Read the model definition and answer for the solid it produces. Units are mm, in the model's axes. Face numbers are marked on the shaded views. A direction names the side the tool comes from. Coordinates: 2 decimals unless noted, no trailing zeros. Order: outer loops, then holes, each group sorted by start corner. A loop starts at its lowest first (then second) coordinate and runs counter-clockwise, first axis right, second up.
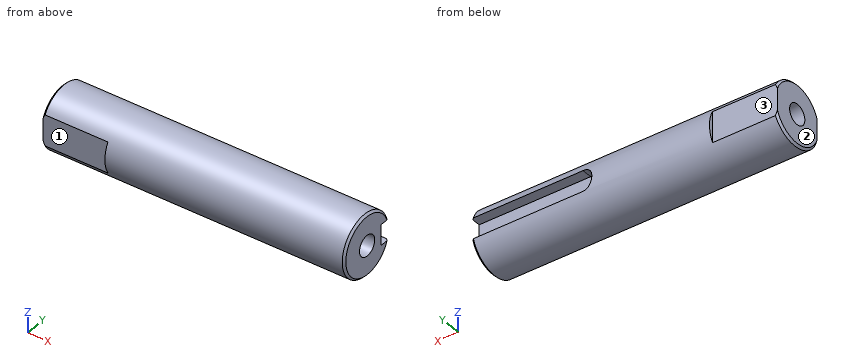
from build123d import *

# Parameters (mm, degrees)
SKETCH_2_W                     = 75
SKETCH_2_H                     = 7.5
CUT_EXTRUDE_START              = 4.5
CUT_EXTRUDE_1_DEPTH            = 72.246287038
CUT_EXTRUDE_2_DEPTH            = 76.746287157
CUT_EXTRUDE_2_DEPTH_BACK       = 76.746287157
SKETCH_4_W                     = 16
SKETCH_4_H                     = 1
M5X0_8_1_D                     = 4.2
M5X0_8_1_DEPTH                 = 14
M5X0_8_1_CBORE_D               = 5
M5X0_8_1_CBORE_DEPTH           = 10
M5X0_8_1_TIP                   = 1.2618073
M5X0_8_1_ON_FACE_2_D           = 4.2
M5X0_8_1_ON_FACE_2_DEPTH       = 14
M5X0_8_1_ON_FACE_2_CBORE_D     = 5
M5X0_8_1_ON_FACE_2_CBORE_DEPTH = 10
M5X0_8_1_ON_FACE_2_TIP         = 1.2618073
CHAMFER_1_SIZE                 = 0.5


with BuildPart() as part:
    # ｽｹｯﾁ2 → 回転1 (revolve)
    with BuildSketch(Plane.XY, mode=Mode.PRIVATE) as revolve_1_sk:
        with Locations((37.5, 3.75)):
            Rectangle(SKETCH_2_W, SKETCH_2_H)
    revolve(revolve_1_sk.sketch.rotate(Axis((0, 0, 0), (1, 0, 0)), 90), axis=Axis((0, 0, 0), (1, 0, 0)))

    # ｽｹｯﾁ3 → ｶｯﾄ - 押し出し1 (cut, through all)
    with BuildSketch(Plane(origin=(0, 0, 0), x_dir=(1, 0, 0), z_dir=(0, 1, 0)).offset(CUT_EXTRUDE_START)):
        with BuildLine():
            Line((47.5, 2.5), (75, 2.5))
            Line((75, 2.5), (75, -2.5))
            Line((75, -2.5), (47.5, -2.5))
            ThreePointArc((47.5, -2.5), (45, 0), (47.5, 2.5))
        make_face()
    extrude(amount=CUT_EXTRUDE_1_DEPTH, mode=Mode.SUBTRACT)

    # ｽｹｯﾁ4 → ｶｯﾄ - 押し出し2 (cut, two sides: drawn at the far end of the back side and taken through both)
    with BuildSketch(Plane.XY.offset(-CUT_EXTRUDE_2_DEPTH_BACK)):
        with Locations((8, 7)):
            Rectangle(SKETCH_4_W, SKETCH_4_H)
        with Locations((8, -7)):
            Rectangle(SKETCH_4_W, SKETCH_4_H)
    extrude(amount=CUT_EXTRUDE_2_DEPTH + CUT_EXTRUDE_2_DEPTH_BACK, mode=Mode.SUBTRACT)

    # M5x0.8 ねじ穴1
    with Locations(Plane(origin=(0, 0, 0), x_dir=(0, 0, -1), z_dir=(-1, 0, 0))):
        with Locations((0, 0)):
            CounterBoreHole(M5X0_8_1_D / 2, M5X0_8_1_CBORE_D / 2, M5X0_8_1_CBORE_DEPTH, depth=M5X0_8_1_DEPTH)
            with Locations((0, 0, -(M5X0_8_1_DEPTH + M5X0_8_1_TIP / 2))):  # 118° drill point
                Cone(0, M5X0_8_1_D / 2, M5X0_8_1_TIP, mode=Mode.SUBTRACT)

    # M5x0.8 ねじ穴1 on face 2
    with Locations(Plane(origin=(75, 0, 0), x_dir=(0, 0, 1), z_dir=(1, 0, 0))):
        with Locations((0, 0)):
            CounterBoreHole(M5X0_8_1_ON_FACE_2_D / 2, M5X0_8_1_ON_FACE_2_CBORE_D / 2, M5X0_8_1_ON_FACE_2_CBORE_DEPTH, depth=M5X0_8_1_ON_FACE_2_DEPTH)
            with Locations((0, 0, -(M5X0_8_1_ON_FACE_2_DEPTH + M5X0_8_1_ON_FACE_2_TIP / 2))):  # 118° drill point
                Cone(0, M5X0_8_1_ON_FACE_2_D / 2, M5X0_8_1_ON_FACE_2_TIP, mode=Mode.SUBTRACT)

    # 面取り1
    chamfer_1_edges = [part.edges().sort_by_distance(p)[0] for p in [
        (0, 0, -7.5),
        (0, -3.754168989, 6.492781777),
        (75, -6.123724357, -4.330127019),
    ]]
    chamfer(chamfer_1_edges, length=CHAMFER_1_SIZE)


solid = part.part
Q1. The part is cut by section A-A, the plane x = 68. Determine the outline of the cut face in (y, z).
Q2. The part is cut by section B-B, the plane x = 54. Determine the outline of the cut face in (y, z).
Q3. Each of these flat-tipped pins is pushed along its axis until it touches: P1, Ø3, axis at x = 59.5, y = 6, coming from the -Z side; P2, Ø1.5, axis at x = 61, y = 5, coming from the -Z side; P3, Ø4.5, axis at y = 0, z = 0, coming from the +X side. Where does it stop, or does it pass through?
Q4. Straight lines are drawn through the part: L1, parallel to Y at x = 71.75, z = 0; L2, parallel to Y at x = 63.3, z = 0; L3, parallel to Z at x = 66, y = 1.75. For each, find the intervals that lie inside material, in ascending order.
Q5. Which of the six approach directions +Z, -Z, +X, -X, +Y, -Y give full straight-line access (tool end or side, diameter ignored) to the marked faces 1, 2 and 3?
Computed values:
1. outline: (4.5, -2.5) - (4.5, 2.5) - (7.07, 2.5) arc R7.5 ccw (long way) to (7.07, -2.5) - close; hole circle Ø5 at (0, 0)
2. outline: (4.5, -2.5) - (4.5, 2.5) - (7.07, 2.5) arc R7.5 ccw (long way) to (7.07, -2.5) - close
3. P1: stops at z = -6
3. P2: stops at z = -6.18
3. P3: stops at x = 65
4. L1: y = -7.5 to -2.5, 2.5 to 4.5
4. L2: y = -7.5 to -2.1, 2.1 to 4.5
4. L3: z = -7.29 to -1.79, 1.79 to 7.29
5. face 1: +Z, -Z, -X, -Y
5. face 2: +Z, -Z, -X, +Y, -Y
5. face 3: +Z, -Z, -X, +Y
